Work out the finished part from the listing and answer in its coordinate system (mm). A direction names the side the tool comes from. Round coordinates to 2 decimals unless told otherwise and drop trailing zeros. Write each loop counter-clockwise with the first axis right and the second up, starting at its lowest first coordinate (ties: lowest second). Pieces come first, ordered by that corner, then holes.
1. Determine the mould class of faces 1 (the face through (0, 0.809, 1.6)), 2 (the face through (-1, 1, -5)), 3 (the face through (-2, -4.191, 5)) for opening direction Z: pulls with the +Z half, pulls with the -Z half, needs draft (parallel to the pull), parting line crosses it, or undercut.
2. Find section D-D (y = -0.75). Write down the section's boundary in (x, z).
3. Straight lines are drawn through the part: probe 1 along Y at (x, z) = (0, 7.9); probe 2 along Z at (x, y) = (-10, 4); probe 3 along X at (y, z) = (3.5, -3.25). For each, find the intervals that lie inside material, in ascending order.
4. A tool of negligible diameter and unlimited length cuts with its end or side. For faces 4 (the face through (0.75, 5, 2)), 5 (the face through (-1.34, 4.42, -2.46)), 6 (the face through (1.13, 2.36, 8.55)), from which of +Z, -Z, +X, -X, +Y, -Y can it reach the whole face along a straight path? Write none if from no direction.
5. Find section B-B (z = 1.5). Write down the section's boundary in (x, y), and give its area (3 significant figures).
6. Find section A-A (x = 0). Write down the section's boundary in (y, z).
7. Find section C-C (y = -2.5). Write down the section's boundary in (x, z), and give its area (3 significant figures).
8. Flat-ended cylindrical pins translate along their axes: pin 1 Ø4 at (x, z) = (0, 4.74) entering from +Y; pin 2 Ø3.5 at (x, y) = (0, 2.31) entering from +Z; pin 3 Ø2 at (x, y) = (0, 2.31) entering from -Z. Find the tip coordinate at first contact, or state that the pin passes through.
```python
from build123d import *

# Parameters (mm, degrees)
SKETCH1_W                = 30
SKETCH1_H                = 10
BOSS_EXTRUDE1_DEPTH      = 10
SKETCH2_R                = 2.5
SKETCH2_R_2              = 1.1303
F_4_40_SCREW_SPACE_DEPTH = 5
SKETCH5_R                = 1.1303
CUT_EXTRUDE3_DEPTH       = 16
SKETCH3_R                = 2.65
CUT_EXTRUDE1_DEPTH       = 8
SKETCH4_W                = 1.5
SKETCH4_H                = 1.778161356
CUT_EXTRUDE2_DEPTH       = 5


with BuildPart() as part:
    # Sketch1 → Boss-Extrude1 (new body)
    with BuildSketch(Plane.XY):
        with Locations((-1.440677966, 0.809495308)):
            Rectangle(SKETCH1_W, SKETCH1_H)
    extrude(amount=BOSS_EXTRUDE1_DEPTH)

    # Sketch2 → 4-40 screw space (add)
    with BuildSketch(Plane(origin=(0, 0, 0), x_dir=(-1, 0, 0), z_dir=(0, 0, -1))):
        with Locations((0, 2.309495308)):
            Circle(SKETCH2_R)
        with Locations((0, 2.309495308)):
            Circle(SKETCH2_R_2, mode=Mode.SUBTRACT)
    extrude(amount=F_4_40_SCREW_SPACE_DEPTH)

    # Sketch5 → Cut-Extrude3 (cut, through all)
    with BuildSketch(Plane(origin=(0, 0, -5), x_dir=(-1, 0, 0), z_dir=(0, 0, -1))):
        with Locations((0, 2.309495308)):
            Circle(SKETCH5_R)
    extrude(amount=-CUT_EXTRUDE3_DEPTH, mode=Mode.SUBTRACT)

    # Sketch3 → Cut-Extrude1 (cut)
    with BuildSketch(Plane(origin=(0, 5.809495308, 0), x_dir=(1, 0, 0), z_dir=(0, 1, 0))):
        with Locations((0, -4.740342164)):
            Circle(SKETCH3_R)
    extrude(amount=-CUT_EXTRUDE1_DEPTH, mode=Mode.SUBTRACT)

    # Sketch4 → Cut-Extrude2 (cut)
    with BuildSketch(Plane(origin=(0, 5.809495308, 0), x_dir=(1, 0, 0), z_dir=(0, 1, 0))):
        with Locations((0, -1.889080678)):
            Rectangle(SKETCH4_W, SKETCH4_H)
    extrude(amount=-CUT_EXTRUDE2_DEPTH, mode=Mode.SUBTRACT)


solid = part.part
```
Worked answers:
1. face 1: undercut
1. face 2: pulls with the -Z half
1. face 3: needs draft
2. outline: (-16.44, 0) - (13.56, 0) - (13.56, 10) - (-16.44, 10) - close; hole circle Ø5.3 at (0, 4.74)
3. probe 1: y = -4.19 to 1.18, 3.44 to 5.81
3. probe 2: z = 0 to 10
3. probe 3: x = -2.2 to 2.2
4. face 4: +Y
4. face 5: -Z
4. face 6: +Z, -Z
5. outline: (-16.44, -4.19) - (13.56, -4.19) - (13.56, 5.81) - (0.75, 5.81) - (0.75, 3.16) arc R1.13 cw to (0.75, 1.46) - (0.75, 0.81) - (-0.75, 0.81) - (-0.75, 1.46) arc R1.13 cw to (-0.75, 3.16) - (-0.75, 5.81) - (-16.44, 5.81) - close
5. area: 292 mm2
6. outline: (-4.19, 0) - (-0.19, 0) - (-0.19, -5) - (1.18, -5) - (1.18, 1) - (0.81, 1) - (0.81, 2.09) - (-2.19, 2.09) - (-2.19, 7.39) - (1.18, 7.39) - (1.18, 10) - (-4.19, 10) - close; (3.44, -5) - (4.81, -5) - (4.81, 0) - (5.81, 0) - (5.81, 1) - (3.44, 1) - close; (3.44, 7.39) - (5.81, 7.39) - (5.81, 10) - (3.44, 10) - close
7. outline: (-16.44, 0) - (13.56, 0) - (13.56, 10) - (-16.44, 10) - close
7. area: 300 mm2
8. pin 1: stops at y = -2.19
8. pin 2: stops at z = 10
8. pin 3: passes through
